Verification items for the finished model (mm, model axes). A direction names the side the tool comes from. Coordinates: 2 decimals unless noted, no trailing zeros. Write each loop counter-clockwise with the first axis right and the second up, starting at its lowest first coordinate (ties: lowest second). Pieces come first, ordered by that corner, then holes. Notation, with made-up numbers: (54, 58.5) -> (81, 58.5) arc R26 cw to (81, 86.5) -> close; hole circle Ø9 at (57, 35). An arc over 180 degrees is marked (long way). Write item = value, one per line. Start each with the question number.
(1) Material ranges on probe 1 along Y at (x, z) = (126, -63) (3 decimals); probe 2 along Z at (x, y) = (-114.3, 1); probe 3 along Z at (x, y) = (63.5, 2.25), recorded low to high. Write a range as [from, to].
(2) Gauge pin test, flat ends, axial feed: pin 1 Ø5 at (x, z) = (38.5, 1.5) entering from +Y (3 decimals); pin 2 Ø4 at (x, z) = (-70.5, 33) entering from -Y; pin 3 Ø2.5 at (x, y) = (-169.5, 2) entering from +Z; pin 4 Ø8 at (x, z) = (-139.7, -12.7) entering from -Y. Record the tip position at first contact, or that the pin passes through.
(3) Section check B-B (z = -29). Record the cut outline in (x, y) (3 decimals).
(4) Section check A-A (x = 44). Record the cut outline in (y, z) (3 decimals), plus the area to 3 significant figures.
(5) Set-up check for faces 1 (the face through (-152.4, -26, 28)), 2 (the face through (2, 3.175, -50)), 3 (the face through (152.4, -26, 28)), 4 (the face through (2, 0, -50)): record each of +Z, -Z, +X, -X, +Y, -Y from which the full face is reachable in a straight line by a thin tool's end or side.
(6) Section check C-C (y = -13.5). Record the cut outline in (x, z), plus the area to 3 significant figures.
```python
from build123d import *

# Parameters (mm, degrees)
SKETCH1_W                      = 101.6
SKETCH1_H                      = 3.175
INITIAL_MIDPLANE_EXTRUDE_DEPTH = 152.4
SKETCH1_3_W                    = 101.6
SKETCH1_3_H                    = 3.175
REEXTRUDE_FOR_WINGS_DEPTH      = 177.8
SKETCH2_W                      = 25.4
SKETCH2_H                      = 25.4
BANDSAW_CUT_DEPTH              = 76.017048969
SKETCH3_R                      = 2.54
INITIAL_MOUNTING_HOLE_DEPTH    = 76.017048969
MOUNTING_HOLE_PATTERN_COUNT    = 12
MOUNTING_HOLE_PATTERN_PITCH    = 25.4


with BuildPart() as part:
    # Sketch1 → Initial MidPlane Extrude (new body, symmetric)
    with BuildSketch(Plane(origin=(0, 0, 0), x_dir=(0, 0, -1), z_dir=(1, 0, 0))):
        with Locations((50.8, 1.5875)):
            Rectangle(SKETCH1_W, SKETCH1_H)
        with BuildLine():
            Line((-71.842048969, -71.842048969), (0, 0))
            Line((0, 0), (0, 3.175))
            ThreePointArc((0, 3.175), (-1.215019898, 2.933317516), (-2.24506403, 2.24506403))
            Line((-2.24506403, 2.24506403), (-74.087112999, -69.596984938))
            Line((-74.087112999, -69.596984938), (-71.842048969, -71.842048969))
        make_face()
    extrude(amount=INITIAL_MIDPLANE_EXTRUDE_DEPTH, both=True)

    # Sketch1_3 → ReExtrude For Wings (add, symmetric)
    with BuildSketch(Plane(origin=(0, 0, 0), x_dir=(0, 0, -1), z_dir=(1, 0, 0))):
        with Locations((50.8, 1.5875)):
            Rectangle(SKETCH1_3_W, SKETCH1_3_H)
    extrude(amount=REEXTRUDE_FOR_WINGS_DEPTH, both=True)

    # Sketch2 → Bandsaw Cut (cut, through all)
    with BuildSketch(Plane(origin=(0, 3.175, 0), x_dir=(1, 0, 0), z_dir=(0, 1, 0))):
        with Locations((-165.1, 12.7)):
            Rectangle(SKETCH2_W, SKETCH2_H)
        with Locations((165.1, 12.7)):
            Rectangle(SKETCH2_W, SKETCH2_H)
    extrude(amount=-BANDSAW_CUT_DEPTH, mode=Mode.SUBTRACT)

    # Sketch3 → Initial Mounting Hole (cut, through all)
    with BuildSketch(Plane(origin=(0, 3.175, 0), x_dir=(1, 0, 0), z_dir=(0, 1, 0))):
        with Locations((-139.7, 12.7)):
            Circle(SKETCH3_R)
    initial_mounting_hole = extrude(amount=-INITIAL_MOUNTING_HOLE_DEPTH, mode=Mode.SUBTRACT)

    # Mounting Hole Pattern: Initial Mounting Hole ×12
    with Locations(*[(i * MOUNTING_HOLE_PATTERN_PITCH, 0, 0) for i in range(1, MOUNTING_HOLE_PATTERN_COUNT)]):
        add(initial_mounting_hole, mode=Mode.SUBTRACT)


solid = part.part
```
Response:
q1.probe_1 = [0, 3.175]
q1.probe_2 = [-101.6, -15.24], [-10.16, 3.49]
q1.probe_3 = [-101.6, -15.24], [-10.16, 2.24]
q2.pin_1 = 3.175
q2.pin_2 = -35
q2.pin_3 = -25.4
q2.pin_4 = 0
q3.outline = (-177.8, 0) -> (177.8, 0) -> (177.8, 3.175) -> (-177.8, 3.175) -> close
q4.outline = (-71.842, 71.842) -> (0, 0) -> (0, -101.6) -> (3.175, -101.6) -> (3.175, 0) arc R3.175 ccw to (2.245, 2.245) -> (-69.597, 74.087) -> close
q4.area = 649 mm2
q5.face_1 = +Z, -X, +Y, -Y
q5.face_2 = +Z, -Z, +X, -X, +Y
q5.face_3 = +Z, +X, +Y, -Y
q5.face_4 = -Z, +X, -X, -Y
q6.outline = (-152.4, 13.5) -> (152.4, 13.5) -> (152.4, 17.99) -> (-152.4, 17.99) -> close
q6.area = 1,370 mm2
